The listing builds one solid part. Answer for the finished solid, in the listing's coordinates (mm). Face numbers are marked on the shaded views. A direction names the side the tool comes from. Coordinates: 2 decimals unless noted, no trailing zeros. Loops run counter-clockwise (first coordinate to the right, second up) from the corner with the lowest first, then second, coordinate; pieces in that order, holes last. Notation, with made-up numbers: (61, 56.5) - (89, 56.5) arc R13 ccw to (89, 73.5) - close; hole circle Ø8 at (48, 34). An arc over 180 degrees is marked (long way). Write each question's results on one line, items separated by ' | '. Start each with the question number.
(1) Find section B-B on y = 6.5. Determine the outline of the cut face in (x, z), then the cut area to 3 significant figures.
(2) Find section D-D on x = -2.25. Determine the outline of the cut face in (y, z), then the cut area to 3 significant figures.
(3) Consider line 1 (X direction, y = 7, z = 5); line 2 (Y direction, x = 0.25, z = 2.5); line 3 (Y direction, x = 4, z = 3.81). Determine where each line is inside the solid, lowest interval first. Write a range as from..to.
(4) For the marked faces 1 and 2, determine the directions among +Z, -Z, +X, -X, +Y, -Y from which every point of the face is accessible in a straight line to the end or side of a thin tool.
(5) Find section C-C on z = 6.25. Determine the outline of the cut face in (x, y).
(6) Find section A-A on z = 3.81. Determine the outline of the cut face in (x, y).
(7) Determine the mould class of the marked faces 3, 4 and 5 for opening direction X: released by +X, released by -X, zero draft, split by the parting line, or undercut.
(8) Given pin 1 Ø1.9 at (x, z) = (1, 2.5) entering from +Y; pin 2 Ø2 at (x, z) = (0, 3) entering from -Y, each flat-ended and moving along its own axis, determine where each tip first touches the part or whether it passes through.
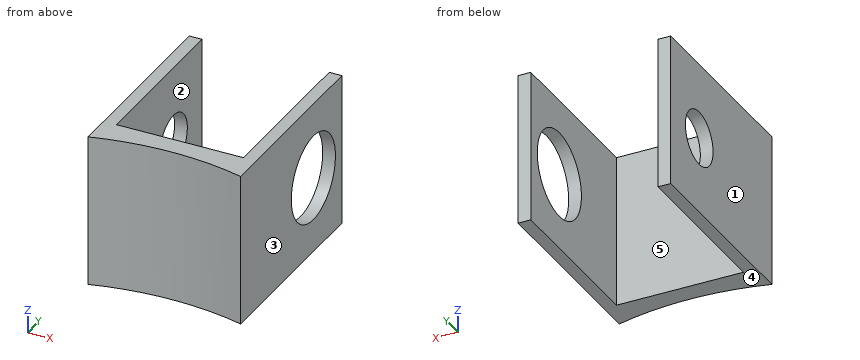
from build123d import *

# Parameters (mm, degrees)
BOSS_EXTRUDE1_DEPTH       = 7.62
F_6_32_TAPPED_HOLE1_D     = 2.7051
F_6_32_TAPPED_HOLE1_DEPTH = 0.635
CUT_EXTRUDE1_REACH        = 9.62
SKETCH6_R                 = 2.159
CUT_EXTRUDE2_DEPTH        = 8.62


with BuildPart() as part:
    # Sketch1 → Boss-Extrude1 (new body)
    with BuildSketch(Plane.XY):
        Polygon((-3.353873239, 7.61418662), (-3.353873239, -2.29181338), (4.266126761, -2.29181338), (4.266126761, 7.61418662), (3.631126761, 7.61418662), (3.631126761, -0.76781338), (-2.718873239, -0.76781338), (-2.718873239, 7.61418662), align=None)
    extrude(amount=BOSS_EXTRUDE1_DEPTH)

    # #6-32 Tapped Hole1
    with Locations(Plane.ZY.offset(3.353873239)):
        with Locations((3.81, 4.82018662)):
            Hole(F_6_32_TAPPED_HOLE1_D / 2, depth=F_6_32_TAPPED_HOLE1_DEPTH)

    # Sketch6 → Cut-Extrude1 (cut, up to next)
    with BuildSketch(Plane(origin=(4.266126761, 0, 0), x_dir=(0, 0, -1), z_dir=(1, 0, 0)), mode=Mode.PRIVATE) as cut_extrude1_sk1:
        with Locations((-3.81, 4.82018662)):
            Circle(SKETCH6_R)
    cut_extrude1_tool1 = extrude(cut_extrude1_sk1.sketch, amount=-CUT_EXTRUDE1_REACH, mode=Mode.PRIVATE) & part.part
    add(cut_extrude1_tool1.solids().sort_by_distance((4.266127, 4.820187, 3.81))[0], mode=Mode.SUBTRACT)

    # Sketch16 → Cut-Extrude2 (cut, through all)
    with BuildSketch(Plane(origin=(0, 0, 0), x_dir=(-1, 0, 0), z_dir=(0, 0, -1))):
        with BuildLine():
            Line((3.353873239, -2.29181338), (-4.266126761, -2.29181338))
            ThreePointArc((-4.266126761, -2.29181338), (-0.456126761, -1.781504099), (3.353873239, -2.29181338))
        make_face()
    extrude(amount=-CUT_EXTRUDE2_DEPTH, mode=Mode.SUBTRACT)


solid = part.part
Values:
1) outline: (-3.35, 0) - (-2.72, 0) - (-2.72, 7.62) - (-3.35, 7.62) - close; (3.63, 0) - (4.27, 0) - (4.27, 2.45) - (3.63, 2.45) - close; (3.63, 5.17) - (4.27, 5.17) - (4.27, 7.62) - (3.63, 7.62) - close | area: 7.95 mm²
2) outline: (-2.04, 0) - (-0.77, 0) - (-0.77, 7.62) - (-2.04, 7.62) - close | area: 9.67 mm²
3) line 1: x = -3.35..-2.72, 3.63..4.27 | line 2: y = -1.78..-0.77 | line 3: y = -2.22..2.66, 6.98..7.61
4) face 1: +Z, -Z, -X, +Y, -Y | face 2: +Z, -Z, +Y
5) outline: (-3.35, -2.29) arc R14.48 cw to (4.27, -2.29) - (4.27, 7.61) - (3.63, 7.61) - (3.63, -0.77) - (-2.72, -0.77) - (-2.72, 7.61) - (-3.35, 7.61) - close
6) outline: (-3.35, -2.29) arc R14.48 cw to (4.27, -2.29) - (4.27, 2.66) - (3.63, 2.66) - (3.63, -0.77) - (-2.72, -0.77) - (-2.72, 3.47) - (-3.35, 3.47) - close; (-3.35, 6.17) - (-2.72, 6.17) - (-2.72, 7.61) - (-3.35, 7.61) - close; (3.63, 6.98) - (4.27, 6.98) - (4.27, 7.61) - (3.63, 7.61) - close
7) face 3: released by +X | face 4: zero draft | face 5: undercut
8) pin 1: stops at y = -0.77 | pin 2: stops at y = -1.85
